Design review of the part built by this model. Coordinates are the model's own, in mm. A direction names the side the tool comes from. Give positions to 0.01 mm unless a question says otherwise; leave off trailing zeros. Loops run counter-clockwise (first coordinate to the right, second up) from the corner with the lowest first, then second, coordinate; pieces in that order, holes last. Notation, with made-up numbers: M 70.25,-38.5 L 104.25,-38.5 A22 ccw 104.25,-4.5 Z; hole C 2.25,31 d1. An arc over 180 degrees is marked long. Use a Markdown table: item, result. Add a question column.
(1) For faces 4 (the face through (10.806, 3.042, 50.836)), 5 (the face through (10.405, 4.93, 46.859)), 6 (the face through (38.623, 3.042, -34.776)), list the 3-axis set-ups (+Z, -Z, +X, -X, +Y, -Y) from which the entire face can be reached by the end or side of a thin tool; tool diameter is ignored.
(2) Insertion check: pin 1 Ø4 at (x, y) = (-36.5, 6) entering from +Z; pin 2 Ø4.5 at (x, z) = (45, -27) entering from +Y; pin 3 Ø3 at (x, y) = (-20.5, 16.5) entering from -Z. Each pin has a flat end and moves straight along its axis. Give the tip position at first contact, or say it passes through.
(3) For probe 1 along X at (y, z) = (16, 0); probe 2 along X at (y, z) = (18.75, 0), list the stretches that pass through material, from the lowest coordinate up.
(4) Draft analysis for pull direction Y (two halves, no side actions). For faces 1 (the face through (-26.34, 29.52, -41.32)), 2 (the face through (43, 0, -24)), 3 (the face through (-40, 17, 25)), state which applies: pulls with the +Y half, pulls with the -Y half, needs draft (parallel to the pull), parting line crosses it, or undercut.
(5) Add section B-B, the plane y = 26.5. Give the boundary of the cut face in (x, z), then the cut area to 3 significant figures.
```python
from build123d import *

# Parameters (mm, degrees)
CUT_EXTRUDE1_DEPTH                  = 6
CUT_EXTRUDE2_DEPTH                  = 6
CUT_EXTRUDE3_DEPTH                  = 6
BOSS_EXTRUDE1_START                 = -6
BOSS_EXTRUDE1_DEPTH                 = 6
BOSS_EXTRUDE2_START                 = -6
BOSS_EXTRUDE2_DEPTH                 = 6
BOSS_EXTRUDE3_START                 = -6
BOSS_EXTRUDE3_DEPTH                 = 6
F_1_5MM_DOWEL_HOLE1_D               = 1.5
F_1_5MM_DOWEL_HOLE1_DEPTH           = 3
F_1_5MM_DOWEL_HOLE1_TIP             = 0.450645464
F_1_5MM_DOWEL_HOLE1_ON_FACE_2_D     = 1.5
F_1_5MM_DOWEL_HOLE1_ON_FACE_2_DEPTH = 3
F_1_5MM_DOWEL_HOLE1_ON_FACE_2_TIP   = 0.450645464
F_1_5MM_DOWEL_HOLE1_ON_FACE_3_D     = 1.5
F_1_5MM_DOWEL_HOLE1_ON_FACE_3_DEPTH = 3
F_1_5MM_DOWEL_HOLE1_ON_FACE_3_TIP   = 0.450645464
F_1_5MM_DOWEL_HOLE1_ON_FACE_4_D     = 1.5
F_1_5MM_DOWEL_HOLE1_ON_FACE_4_DEPTH = 3
F_1_5MM_DOWEL_HOLE1_ON_FACE_4_TIP   = 0.450645464
F_1_5MM_DOWEL_HOLE1_ON_FACE_5_D     = 1.5
F_1_5MM_DOWEL_HOLE1_ON_FACE_5_DEPTH = 3
F_1_5MM_DOWEL_HOLE1_ON_FACE_5_TIP   = 0.450645464
F_1_5MM_DOWEL_HOLE1_ON_FACE_6_D     = 1.5
F_1_5MM_DOWEL_HOLE1_ON_FACE_6_DEPTH = 3
F_1_5MM_DOWEL_HOLE1_ON_FACE_6_TIP   = 0.450645464


with BuildPart() as part:
    # Sketch1 → Revolve1 (revolve)
    with BuildSketch(Plane.XY):
        Polygon((-49, 31), (-42, 31), (-42, 6), (-43, 6), (-44, 7), (-44, 10), (-48, 10), (-48, 0), (-50, 0), (-50, 12), (-54, 12), (-54, 14), (-49, 14), (-49, 17), (-47, 17), (-47, 28), (-49, 28), align=None)
    revolve(axis=Axis((0, 15.855614973, 0), (0, -1, 0)))

    # Sketch2 → Cut-Extrude1 (cut)
    with BuildSketch(Plane.XZ):
        with BuildLine():
            Line((10.395584541, -48.907380037), (9.979761159, -46.951084835))
            ThreePointArc((9.979761159, -46.951084835), (0, -48), (-9.979761159, -46.951084835))
            Line((-9.979761159, -46.951084835), (-10.395584541, -48.907380037))
            ThreePointArc((-10.395584541, -48.907380037), (0, -50), (10.395584541, -48.907380037))
        make_face()
    extrude(amount=-CUT_EXTRUDE1_DEPTH, mode=Mode.SUBTRACT)

    # Sketch2_5 → Cut-Extrude2 (cut)
    with BuildSketch(Plane.XZ):
        with BuildLine():
            ThreePointArc((-45.650712782, 14.83281573), (-41.569219382, 24), (-35.670951623, 32.118269105))
            Line((-35.670951623, 32.118269105), (-37.157241274, 33.456530318))
            ThreePointArc((-37.157241274, 33.456530318), (-43.301270189, 25), (-47.552825815, 15.450849719))
            Line((-47.552825815, 15.450849719), (-45.650712782, 14.83281573))
        make_face()
    extrude(amount=-CUT_EXTRUDE2_DEPTH, mode=Mode.SUBTRACT)

    # Sketch2_6 → Cut-Extrude3 (cut)
    with BuildSketch(Plane.XZ):
        with BuildLine():
            Line((37.157241274, 33.456530318), (35.670951623, 32.118269105))
            ThreePointArc((35.670951623, 32.118269105), (41.569219382, 24), (45.650712782, 14.83281573))
            Line((45.650712782, 14.83281573), (47.552825815, 15.450849719))
            ThreePointArc((47.552825815, 15.450849719), (43.301270189, 25), (37.157241274, 33.456530318))
        make_face()
    extrude(amount=-CUT_EXTRUDE3_DEPTH, mode=Mode.SUBTRACT)

    # Sketch2_7 → Boss-Extrude1 (add)
    with BuildSketch(Plane.XZ.offset(BOSS_EXTRUDE1_START)):
        with BuildLine():
            ThreePointArc((47.552825815, -15.450849719), (43.301270189, -25), (37.157241274, -33.456530318))
            Line((37.157241274, -33.456530318), (40.129820576, -36.133052743))
            ThreePointArc((40.129820576, -36.133052743), (46.765371804, -27), (51.35705188, -16.686917696))
            Line((51.35705188, -16.686917696), (47.552825815, -15.450849719))
        make_face()
    extrude(amount=BOSS_EXTRUDE1_DEPTH)

    # Sketch2_8 → Boss-Extrude2 (add)
    with BuildSketch(Plane.XZ.offset(BOSS_EXTRUDE2_START)):
        with BuildLine():
            ThreePointArc((-10.395584541, 48.907380037), (-5.226423163, 49.726094768), (0, 50))
            ThreePointArc((0, 50), (5.226423163, 49.726094768), (10.395584541, 48.907380037))
            Line((10.395584541, 48.907380037), (11.227231304, 52.81997044))
            ThreePointArc((11.227231304, 52.81997044), (0, 54), (-11.227231304, 52.81997044))
            Line((-11.227231304, 52.81997044), (-10.395584541, 48.907380037))
        make_face()
    extrude(amount=BOSS_EXTRUDE2_DEPTH)

    # Sketch2_9 → Boss-Extrude3 (add)
    with BuildSketch(Plane.XZ.offset(BOSS_EXTRUDE3_START)):
        with BuildLine():
            Line((-40.129820576, -36.133052743), (-37.157241274, -33.456530318))
            ThreePointArc((-37.157241274, -33.456530318), (-43.301270189, -25), (-47.552825815, -15.450849719))
            Line((-47.552825815, -15.450849719), (-51.35705188, -16.686917696))
            ThreePointArc((-51.35705188, -16.686917696), (-46.765371804, -27), (-40.129820576, -36.133052743))
        make_face()
    extrude(amount=BOSS_EXTRUDE3_DEPTH)

    # 1.5mm Dowel Hole1
    with Locations(Plane(origin=(6.577263108, 3, 53.597944084), x_dir=(0.992554520069, 0, -0.121801168675), z_dir=(0.121801168675, 0, 0.992554520069))):
        with Locations((0, 0)):
            Hole(F_1_5MM_DOWEL_HOLE1_D / 2, depth=F_1_5MM_DOWEL_HOLE1_DEPTH)
            with Locations((0, 0, -(F_1_5MM_DOWEL_HOLE1_DEPTH + F_1_5MM_DOWEL_HOLE1_TIP / 2))):  # 118° drill point
                Cone(0, F_1_5MM_DOWEL_HOLE1_D / 2, F_1_5MM_DOWEL_HOLE1_TIP, mode=Mode.SUBTRACT)

    # 1.5mm Dowel Hole1 on face 2
    with Locations(Plane(origin=(-6.584625948, 3, 53.597040041), x_dir=(0.992537723435, 0, 0.121937966023), z_dir=(-0.121937966023, 0, 0.992537723435))):
        with Locations((0, 0)):
            Hole(F_1_5MM_DOWEL_HOLE1_ON_FACE_2_D / 2, depth=F_1_5MM_DOWEL_HOLE1_ON_FACE_2_DEPTH)
            with Locations((0, 0, -(F_1_5MM_DOWEL_HOLE1_ON_FACE_2_DEPTH + F_1_5MM_DOWEL_HOLE1_ON_FACE_2_TIP / 2))):  # 118° drill point
                Cone(0, F_1_5MM_DOWEL_HOLE1_ON_FACE_2_D / 2, F_1_5MM_DOWEL_HOLE1_ON_FACE_2_TIP, mode=Mode.SUBTRACT)

    # 1.5mm Dowel Hole1 on face 3
    with Locations(Plane(origin=(-49.705812721, 3, -21.102895103), x_dir=(0.39079405883, 0, -0.920478138569), z_dir=(-0.920478138569, 0, -0.39079405883))):
        with Locations((-1e-09, 0)):
            Hole(F_1_5MM_DOWEL_HOLE1_ON_FACE_3_D / 2, depth=F_1_5MM_DOWEL_HOLE1_ON_FACE_3_DEPTH)
            with Locations((0, 0, -(F_1_5MM_DOWEL_HOLE1_ON_FACE_3_DEPTH + F_1_5MM_DOWEL_HOLE1_ON_FACE_3_TIP / 2))):  # 118° drill point
                Cone(0, F_1_5MM_DOWEL_HOLE1_ON_FACE_3_D / 2, F_1_5MM_DOWEL_HOLE1_ON_FACE_3_TIP, mode=Mode.SUBTRACT)

    # 1.5mm Dowel Hole1 on face 4
    with Locations(Plane(origin=(-43.124085269, 3, -32.500973366), x_dir=(0.601870037997, 0, -0.798594050417), z_dir=(-0.798594050417, 0, -0.601870037997))):
        with Locations((0, 0)):
            Hole(F_1_5MM_DOWEL_HOLE1_ON_FACE_4_D / 2, depth=F_1_5MM_DOWEL_HOLE1_ON_FACE_4_DEPTH)
            with Locations((0, 0, -(F_1_5MM_DOWEL_HOLE1_ON_FACE_4_DEPTH + F_1_5MM_DOWEL_HOLE1_ON_FACE_4_TIP / 2))):  # 118° drill point
                Cone(0, F_1_5MM_DOWEL_HOLE1_ON_FACE_4_D / 2, F_1_5MM_DOWEL_HOLE1_ON_FACE_4_TIP, mode=Mode.SUBTRACT)

    # 1.5mm Dowel Hole1 on face 5
    with Locations(Plane(origin=(43.128549613, 3, -32.495048981), x_dir=(0.601759985579, 0, 0.79867698086), z_dir=(0.79867698086, 0, -0.601759985579))):
        with Locations((0, 0)):
            Hole(F_1_5MM_DOWEL_HOLE1_ON_FACE_5_D / 2, depth=F_1_5MM_DOWEL_HOLE1_ON_FACE_5_DEPTH)
            with Locations((0, 0, -(F_1_5MM_DOWEL_HOLE1_ON_FACE_5_DEPTH + F_1_5MM_DOWEL_HOLE1_ON_FACE_5_TIP / 2))):  # 118° drill point
                Cone(0, F_1_5MM_DOWEL_HOLE1_ON_FACE_5_D / 2, F_1_5MM_DOWEL_HOLE1_ON_FACE_5_TIP, mode=Mode.SUBTRACT)

    # 1.5mm Dowel Hole1 on face 6
    with Locations(Plane(origin=(49.708711217, 3, -21.096066675), x_dir=(0.39066787318, 0, 0.920531701173), z_dir=(0.920531701173, 0, -0.39066787318))):
        with Locations((0, 0)):
            Hole(F_1_5MM_DOWEL_HOLE1_ON_FACE_6_D / 2, depth=F_1_5MM_DOWEL_HOLE1_ON_FACE_6_DEPTH)
            with Locations((0, 0, -(F_1_5MM_DOWEL_HOLE1_ON_FACE_6_DEPTH + F_1_5MM_DOWEL_HOLE1_ON_FACE_6_TIP / 2))):  # 118° drill point
                Cone(0, F_1_5MM_DOWEL_HOLE1_ON_FACE_6_D / 2, F_1_5MM_DOWEL_HOLE1_ON_FACE_6_TIP, mode=Mode.SUBTRACT)


solid = part.part
```
Established:
| question | item | result |
|---|---|---|
| 1 | face 4 | +X, -Y |
| 1 | face 5 | -Y |
| 1 | face 6 | -Z, -Y |
| 2 | pin 1 | z = 36.19 |
| 2 | pin 2 | y = 14 |
| 2 | pin 3 | z = -45.17 |
| 3 | probe 1 | -49 to -42, 42 to 49 |
| 3 | probe 2 | -47 to -42, 42 to 47 |
| 4 | face 1 | needs draft |
| 4 | face 2 | pulls with the -Y half |
| 4 | face 3 | undercut |
| 5 | outline | C 0,0 d94; hole C 0,0 d84 |
| 5 | area | 1,400 mm^2 |
